from build123d import *

# Parameters (mm, degrees)
F1_DEPTH    = 8
F2_R        = 1.5
F3_DEPTH    = 8
F4_DEPTH    = 2
F5_SIZE2    = 5
F5_SIZE     = 37
F6_T1_DEPTH = 198.6904330104


# Not quite as in the source:
# - a fillet or chamfer that OpenCascade refuses, or shapes differently, is made with other operations: its cross-section is extruded or revolved along the edge and cut away or added


with BuildPart() as f1:
    # F0 (on Top) → F1 (new body)
    with BuildSketch(Plane.XY):
        Polygon((0, -4), (40, -4), (75, 31), (63.686291501, 31), (36.686291501, 4), (0, 4), align=None)
    extrude(amount=F1_DEPTH)

    # F2 (on face) → F3 (cut, through all)
    with BuildSketch(Plane(origin=(0, 4, 0), x_dir=(-1, 0, 0), z_dir=(0, 1, 0))):
        with Locations((-30, 4)):
            Circle(F2_R)
    extrude(amount=-F3_DEPTH, mode=Mode.SUBTRACT)

    # F2 (on face) → F4 (cut)
    with BuildSketch(Plane(origin=(0, 4, 0), x_dir=(-1, 0, 0), z_dir=(0, 1, 0))):
        Polygon((-28.4122867597, 1.25), (-26.8245735195, 4), (-28.4122867597, 6.75), (-31.5877132403, 6.75), (-33.1754264805, 4), (-31.5877132403, 1.25), align=None)
        with Locations((-30, 4)):
            Circle(F2_R, mode=Mode.SUBTRACT)
    extrude(amount=-F4_DEPTH, mode=Mode.SUBTRACT)

    # F5
    f5_edges = [f1.edges().sort_by_distance(p)[0] for p in [
        (63.686292, 31, 4),
    ]]
    f5_side = f1.faces().sort_by_distance((50.186292, 17.5, 4))[0]
    chamfer(f5_edges, length=F5_SIZE, length2=F5_SIZE2, reference=f5_side)

    # F6: chamfer of 37 x 3 on 2 edges, made by hand

    # F6_s2 → F6_t1 (cut)
    with BuildSketch(Plane.YZ.offset(-27.5020707547)):
        Polygon((-6, 0), (31, 3), (31, 0), align=None)
        Polygon((31, 5), (-6, 8), (31, 8), align=None)
    extrude(amount=F6_T1_DEPTH, mode=Mode.SUBTRACT)

    # F7: F1 across plane


with BuildPart() as f1_1:
    add(f1.part)
    add(f1.part.mirror(Plane.YZ))


solid = f1_1.part
The model under review builds one solid part; all positions refer to its coordinate system, in mm. A direction names the side the tool comes from. Coordinates: 2 decimals unless noted, no trailing zeros. Order: outer loops, then holes, each group sorted by start corner. A loop starts at its lowest first (then second) coordinate and runs counter-clockwise, first axis right, second up. Notation, with made-up numbers: (78.5, -37.75) -> (92.5, -37.75) arc R15 ccw to (92.5, -30.75) -> close; hole circle Ø9 at (49.5, 82). An arc over 180 degrees is marked (long way). Answer in a Markdown table with one row per item.
(1) Consider section C-C (x = 66). Write out the cut boundary in (y, z).
Answers:
| item | result |
|---|---|
| outline | (22, 2.27) -> (28.74, 2.82) -> (28.74, 5.18) -> (22, 5.73) -> close |
(2) Consider section A-A (x = 30). Write out the cut boundary in (y, z), plus the area to 3 significant figures.
Answers:
| item | result |
|---|---|
| outline | (-4, 0.16) -> (4, 0.81) -> (4, 1.25) -> (2, 1.25) -> (2, 2.5) -> (-4, 2.5) -> close; (-4, 5.5) -> (2, 5.5) -> (2, 6.75) -> (4, 6.75) -> (4, 7.19) -> (-4, 7.84) -> close |
| area | 27.2 mm² |
(3) Wall thickness on line 1 along Y through (x, z) = (27, 6); line 2 along Z through (x, y) = (-30, -2.55); line 3 along Z through (x, y) = (-30, 0.2): over which ranges is each line inside the solid? List them lowest first.
Answers:
| item | result |
|---|---|
| line 1 | -4 to 4 |
| line 2 | 0.28 to 2.5, 5.5 to 7.72 |
| line 3 | 0.5 to 2.5, 5.5 to 7.5 |
(4) Consider section B-B (y = 13.5). Write out the cut boundary in (x, z), plus the area to 3 significant figures.
Answers:
| item | result |
|---|---|
| outline | (-57.5, 1.58) -> (-47.84, 1.58) -> (-47.84, 6.42) -> (-57.5, 6.42) -> close; (47.84, 1.58) -> (57.5, 1.58) -> (57.5, 6.42) -> (47.84, 6.42) -> close |
| area | 93.4 mm² |
(5) The part is to be moulded in two halves that separate along Z. For faces 1 (the flat face through (-1, 4, 4)), 2 (the flat face through (0.35, 3.211, 7.253)), 3 (the flat face through (28.6, 2, 5.3)), say which applies: +Z half, -Z half, draft (parallel to the pull), parting line (faces both ways), or undercut.
Answers:
| item | result |
|---|---|
| face 1 | draft |
| face 2 | +Z half |
| face 3 | undercut |
(6) Insertion check: pin 1 (1.6 mm diameter, centred on x = -30, y = 3.5, fed in from -Z); pin 2 (8 mm diameter, centred on x = 52, y = 10.5, fed in from -Z); pin 3 (1.6 mm diameter, centred on x = -29.5, z = 2.5, fed in from +Y); pin 4 (4 mm diameter, centred on x = -30, z = 4, fed in from -Y). Each pin has a flat end and moves straight along its axis. Give the tip position at first contact, or say it passes through.
Answers:
| item | result |
|---|---|
| pin 1 | z = 0.71 |
| pin 2 | z = 1.03 |
| pin 3 | y = 2 |
| pin 4 | y = -4 |
(7) Machinability: for faces 4 (the flat face through (49.86, 15.195, 3.956)), 5 (the cylindrical face through (-31.5, -0.96, 4.07)), 6 (the flat face through (-28.6, 2, 5.3)), which of the approach directions +Z, -Z, +X, -X, +Y, -Y give a long, thin tool a straight path to every point of the face, cutting with its end or side? Answer none if there is none.
Answers:
| item | result |
|---|---|
| face 4 | +Z, -Z, +Y |
| face 5 | +Y, -Y |
| face 6 | +Y |
